Solid Edge part; units mm, degrees
sketch "Sketch1" plane through (0, 0, 0) normal (0, 0, 1) x (1, 0, 0)
  circle A0 centre (0, 0) radius 38
  circle A1 centre (0, 0) radius 33
extrude "Protrusion1" add sketch "Sketch1" along normal blind 35
hole "Hole_1" at (-35.5, 0, 0) direction (0, 0, 1) diameter 2.459 depth 15 thread major 3 thread length 2
hole "Hole_2" at (-35.5, 0, 35) direction (0, 0, -1) diameter 2.459 depth 15 thread major 3 thread length 2
pattern_circular "Pattern1" count 6 over 360 about axis through (0, 0, 35) along (0, 0, -1) of "Hole_1", "Hole_2"
The listing builds one solid part. Answer for the finished solid, in the listing's coordinates (mm). A direction names the side the tool comes from. Give positions to 0.01 mm unless a question says otherwise; leave off trailing zeros. Loops run counter-clockwise (first coordinate to the right, second up) from the corner with the lowest first, then second, coordinate; pieces in that order, holes last. Notation, with made-up numbers: M 21.5,64 L 47.5,64 A12 ccw 47.5,74 Z; hole C 64,61 d11. An arc over 180 degrees is marked long. One line per item, written item: value.
Q1. Find the intervals of material crossed by line 1 (Y direction, x = 17, z = 10); line 2 (Y direction, x = -35, z = 9); line 3 (X direction, y = 29, z = 15), in increasing order. Write a range as from..to.
Working result:
line 1: y = -33.99..-31.72, -29.77..-28.28, 28.28..29.77, 31.72..33.99
line 2: y = -14.8..-1.12, 1.12..14.8
line 3: x = -24.56..-15.75, 15.75..24.56
Q2. A cutting plane is placed at B-B on y = -12. Determine the outline of the cut face in (x, z), then the cut area to 3 significant figures.
Working result:
outline: M -36.06,0 L -30.74,0 L -30.74,35 L -36.06,35 Z; M 30.74,0 L 36.06,0 L 36.06,35 L 30.74,35 Z
area: 372 mm^2
Q3. A cutting plane is placed at A-A on x = 0. Determine the outline of the cut face in (y, z), then the cut area to 3 significant figures.
Working result:
outline: M -38,0 L -33,0 L -33,35 L -38,35 Z; M 33,0 L 38,0 L 38,35 L 33,35 Z
area: 350 mm^2
Q4. Determine the mould class of faces 1 (the face through (-11.44, 31.14, 0)), 2 (the face through (-36, 0, 20)), 3 (the face through (17.535, 33.713, 17.255)) for opening direction X: +X half, -X half, draft (parallel to the pull), parting line (faces both ways), or undercut.
Working result:
face 1: draft
face 2: undercut
face 3: parting line
Q5. Flat-ended cylindrical pins translate along their axes: P1, Ø2, axis at x = 17.75, y = -30.74, coming from the +Z side; P2, Ø12, axis at x = -18.5, z = 26, coming from the +Y side; P3, Ø1, axis at y = -28.5, z = 19, coming from the +X side. Find the tip coordinate at first contact, or state that the pin passes through.
Working result:
P1: stops at z = 20
P2: stops at y = 35.89
P3: stops at x = 25.69
Q6. For faces 4 (the face through (-36.72, -0.16, 7.6)), 5 (the face through (-16.71, 31.4, 27.4)), determine the directions among +Z, -Z, +X, -X, +Y, -Y from which every point of the face is accessible in a straight line to the end or side of a thin tool.
Working result:
face 4: -Z
face 5: +Z
Q7. A cutting plane is placed at D-D on x = -35.5. Determine the outline of the cut face in (y, z).
Working result:
outline: M -13.56,0 L -1.23,0 L -1.23,15 L 1.23,15 L 1.23,0 L 13.56,0 L 13.56,35 L 1.23,35 L 1.23,20 L -1.23,20 L -1.23,35 L -13.56,35 Z
Q8. A cutting plane is placed at C-C on z = 16.5. Determine the outline of the cut face in (x, y).
Working result:
outline: C 0,0 d76; hole C 0,0 d66
